Verification items for the finished model (mm, model axes). Face numbers are marked on the shaded views. A direction names the side the tool comes from. Coordinates: 2 decimals unless noted, no trailing zeros. Loops run counter-clockwise (first coordinate to the right, second up) from the corner with the lowest first, then second, coordinate; pieces in that order, holes last.
Q1. Mould release check, pull along Z, two halves, no side actions. Record for the marked faces 4, 5, 6 and 7: +Z half, -Z half, draft (parallel to the pull), parting line (faces both ways), or undercut.
Q2. Sectioned sample at D-D (x = 12). Enter the section's corners in (y, z).
Q3. Go/stop test with flat-tipped pins: P1, Ø14, axis at x = 19.5, z = 12.5, coming from the -Y side; P2, Ø2.5, axis at x = 13, y = 4.5, coming from the +Z side; P3, Ø3, axis at x = 15, z = 14, coming from the -Y side; P4, Ø6, axis at x = 34.43, z = 19.57, coming from the +Y side. Record where each tip stops, or that it passes through.
Q4. Sectioned sample at C-C (z = 2). Enter the section's corners in (x, y).
Q5. Sectioned sample at B-B (x = 34.43). Enter the section's corners in (y, z), then the cut area to 4 significant figures.
Q6. Sectioned sample at A-A (y = 3). Enter the section's corners in (x, z).
Q7. Material ranges on probe 1 along Z at (x, y) = (34.43, -3.5); probe 2 along Y at (x, z) = (30.5, 16.75); probe 3 along Z at (x, y) = (34.5, 8.5), recorded low to high.
Q8. Access from +Z, -Z, +X, -X, +Y, -Y to the whole of each face (thin tool, end or side, straight path). Record for the marked faces 1, 2 and 3.
```python
from build123d import *

# Parameters (mm, degrees)
F0_R     = 3.65
F1_DEPTH = 9.5
F0_W     = 40
F0_H     = 3.34
F2_DEPTH = 12.5
F4_DEPTH = 1.5
F5_W     = 13
F5_H     = 2.5
F6_DEPTH = 40.001


with BuildPart() as f1:
    # F0 (on Front) → F1 (new body, symmetric)
    with BuildSketch(Plane.XZ):
        with BuildLine():
            ThreePointArc((28.86, 19.57), (34.43, 14), (40, 19.57))
            ThreePointArc((40, 19.57), (34.43, 25.14), (28.86, 19.57))
        make_face()
        with Locations((34.43, 19.57)):
            Circle(F0_R, mode=Mode.SUBTRACT)
        with BuildLine():
            Line((40, 3.34), (40, 19.57))
            ThreePointArc((40, 19.57), (34.43, 14), (28.86, 19.57))
            Line((28.86, 19.57), (28.86, 6.68))
            Line((28.86, 6.68), (0, 6.68))
            Line((0, 6.68), (0, 3.34))
            Line((0, 3.34), (40, 3.34))
        make_face()
    extrude(amount=F1_DEPTH, both=True)

    # F0 (on Front) → F2 (join, symmetric)
    with BuildSketch(Plane.XZ):
        with Locations((20, 1.67)):
            Rectangle(F0_W, F0_H)
    extrude(amount=F2_DEPTH, both=True)

    # F3 (on Front) → F4 (join, symmetric)
    with BuildSketch(Plane.XZ):
        with BuildLine():
            ThreePointArc((28.86, 19.57), (29.6248313017, 22.3869582498), (31.7092832247, 24.4303086557))
            Line((31.7092832247, 24.4303086557), (0, 6.68))
            Line((0, 6.68), (28.86, 6.68))
            Line((28.86, 6.68), (28.86, 19.57))
        make_face()
    extrude(amount=F4_DEPTH, both=True)

    # F5 (on face) → F6 (cut, through all)
    with BuildSketch(Plane(origin=(0, 0, 0), x_dir=(0, -1, 0), z_dir=(-1, 0, 0))):
        with Locations((0, 1.25)):
            Rectangle(F5_W, F5_H)
    extrude(amount=-F6_DEPTH, mode=Mode.SUBTRACT)


solid = f1.part
```
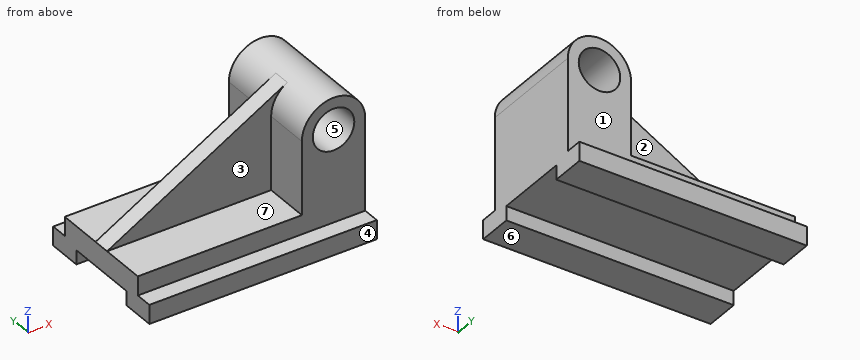
Geometry check:
1. face 4: draft
1. face 5: undercut
1. face 6: -Z half
1. face 7: +Z half
2. outline: (-12.5, 0) - (-6.5, 0) - (-6.5, 2.5) - (6.5, 2.5) - (6.5, 0) - (12.5, 0) - (12.5, 3.34) - (9.5, 3.34) - (9.5, 6.68) - (1.5, 6.68) - (1.5, 13.4) - (-1.5, 13.4) - (-1.5, 6.68) - (-9.5, 6.68) - (-9.5, 3.34) - (-12.5, 3.34) - close
3. P1: stops at y = -9.5
3. P2: stops at z = 6.68
3. P3: stops at y = -1.5
3. P4: passes through
4. outline: (0, -12.5) - (40, -12.5) - (40, -6.5) - (0, -6.5) - close; (0, 6.5) - (40, 6.5) - (40, 12.5) - (0, 12.5) - close
5. outline: (-12.5, 0) - (-6.5, 0) - (-6.5, 2.5) - (6.5, 2.5) - (6.5, 0) - (12.5, 0) - (12.5, 3.34) - (9.5, 3.34) - (9.5, 15.92) - (-9.5, 15.92) - (-9.5, 3.34) - (-12.5, 3.34) - close; (-9.5, 23.22) - (9.5, 23.22) - (9.5, 25.14) - (-9.5, 25.14) - close
5. area: 326.5 mm2
6. outline: (0, 2.5) - (40, 2.5) - (40, 19.57) arc R5.57 ccw to (28.86, 19.57) - (28.86, 6.68) - (0, 6.68) - close; hole circle Ø7.3 at (34.43, 19.57)
7. probe 1: z = 2.5 to 15.92, 23.22 to 25.14
7. probe 2: y = -9.5 to 9.5
7. probe 3: z = 0 to 15.92, 23.22 to 25.14
8. face 1: +Z, +X, -X, +Y
8. face 2: +Z, -X, +Y
8. face 3: +Z, -X, -Y
